Model file for the job. Use its own axes, mm. Coordinates: 2 decimals unless noted, no trailing zeros. Put each result on its own line as item: value. Start each with the question number.
Q1. Drop flat-ended pins along their axis: pin 1 (5.5 mm diameter, centred on x = 184.76, z = -85.27, fed in from +Y); pin 2 (7 mm diameter, centred on x = 306.5, z = -40, fed in from -Y); pin 3 (5.5 mm diameter, centred on x = 182.5, z = -84.5, fed in from -Y). Give the stop position or say it passes through.
Q2. Cut at A-A (y = -11). Give the number of separate pieces and of enclosed holes in the cut face, then the cut area to 3 significant figures.
Q3. Drill centre lines: line 1 along Z through (x, y) = (-194, -12.5); line 2 along X through (y, z) = (-16.75, 65.5); line 3 along X through (y, z) = (-15, 72). Where is each one in solid material? Low to high.
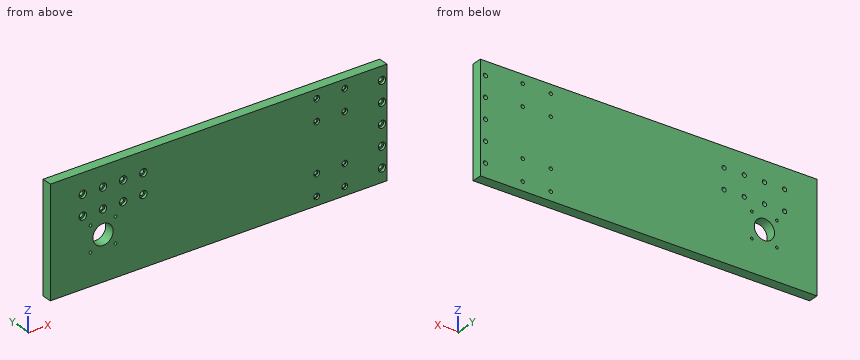
```python
from build123d import *

# Parameters (mm, degrees)
F0_W      = 635
F0_H      = 203.2
F1_DEPTH  = 19.05
F2_R      = 3.99923
F3_DEPTH  = 19.051
F4_R      = 19.05
F4_R_2    = 2.54
F5_DEPTH  = 19.051
F6_R      = 3.175
F7_DEPTH  = 19.051
F8_R      = 3.8735
F9_DEPTH  = 19.051
F10_R     = 6.985
F11_DEPTH = 4.826
F12_R     = 5.461
F13_DEPTH = 3.81


with BuildPart() as f1:
    # F0 (on Front) → F1 (new body)
    with BuildSketch(Plane.XZ):
        Rectangle(F0_W, F0_H)
    extrude(amount=F1_DEPTH)

    # F2 (on face) → F3 (cut, through all)
    with BuildSketch(Plane.XZ.offset(19.05)):
        with Locations((-256.3622, 63.8302)):
            Circle(F2_R)
        with Locations((-218.2622, 63.8302)):
            Circle(F2_R)
        with Locations((-180.1622, 63.8302)):
            Circle(F2_R)
        with Locations((-142.0622, 63.8302)):
            Circle(F2_R)
        with Locations((-142.0622, 25.7302)):
            Circle(F2_R)
        with Locations((-180.1622, 25.7302)):
            Circle(F2_R)
        with Locations((-218.2622, 25.7302)):
            Circle(F2_R)
        with Locations((-256.3622, 25.7302)):
            Circle(F2_R)
    extrude(amount=-F3_DEPTH, mode=Mode.SUBTRACT)

    # F4 (on face) → F5 (cut, through all)
    with BuildSketch(Plane.XZ.offset(19.05)):
        with Locations((-218.2622, -18.7198)):
            Circle(F4_R)
        with Locations((-241.8334, 4.8514)):
            Circle(F4_R_2)
        with Locations((-194.691, 4.8514)):
            Circle(F4_R_2)
        with Locations((-194.691, -42.291)):
            Circle(F4_R_2)
        with Locations((-241.8334, -42.291)):
            Circle(F4_R_2)
    extrude(amount=-F5_DEPTH, mode=Mode.SUBTRACT)

    # F6 (on face) → F7 (cut, through all)
    with BuildSketch(Plane.XZ.offset(19.05)):
        with Locations((184.7596, 85.2678)):
            Circle(F6_R)
        with Locations((237.7694, 85.2678)):
            Circle(F6_R)
        with Locations((184.7596, 45.2628)):
            Circle(F6_R)
        with Locations((237.7694, 45.2628)):
            Circle(F6_R)
        with Locations((184.7596, -45.2628)):
            Circle(F6_R)
        with Locations((237.7694, -45.2628)):
            Circle(F6_R)
        with Locations((184.7596, -85.2678)):
            Circle(F6_R)
        with Locations((237.7694, -85.2678)):
            Circle(F6_R)
    extrude(amount=-F7_DEPTH, mode=Mode.SUBTRACT)

    # F8 (on face) → F9 (cut, through all)
    with BuildSketch(Plane.XZ.offset(19.05)):
        with Locations((307.975, 76.2)):
            Circle(F8_R)
        with Locations((307.975, 38.1)):
            Circle(F8_R)
        with Locations((307.975, 0)):
            Circle(F8_R)
        with Locations((307.975, -38.1)):
            Circle(F8_R)
        with Locations((307.975, -76.2)):
            Circle(F8_R)
    extrude(amount=-F9_DEPTH, mode=Mode.SUBTRACT)

    # F10 (on face) → F11 (cut)
    with BuildSketch(Plane.XZ.offset(19.05)):
        with Locations((-256.3622, 63.8302)):
            Circle(F10_R)
        with Locations((-256.3622, 25.7302)):
            Circle(F10_R)
        with Locations((-218.2622, 25.7302)):
            Circle(F10_R)
        with Locations((-218.2622, 63.8302)):
            Circle(F10_R)
        with Locations((-180.1622, 63.8302)):
            Circle(F10_R)
        with Locations((-142.0622, 63.8302)):
            Circle(F10_R)
        with Locations((-180.1622, 25.7302)):
            Circle(F10_R)
        with Locations((-142.0622, 25.7302)):
            Circle(F10_R)
        with Locations((307.975, -76.2)):
            Circle(F10_R)
        with Locations((307.975, -38.1)):
            Circle(F10_R)
        with Locations((307.975, 0)):
            Circle(F10_R)
        with Locations((307.975, 38.1)):
            Circle(F10_R)
        with Locations((307.975, 76.2)):
            Circle(F10_R)
    extrude(amount=-F11_DEPTH, mode=Mode.SUBTRACT)

    # F12 (on face) → F13 (cut)
    with BuildSketch(Plane.XZ.offset(19.05)):
        with Locations((184.7596, 85.2678)):
            Circle(F12_R)
        with Locations((184.7596, 45.2628)):
            Circle(F12_R)
        with Locations((184.7596, -45.2628)):
            Circle(F12_R)
        with Locations((184.7596, -85.2678)):
            Circle(F12_R)
        with Locations((237.7694, -85.2678)):
            Circle(F12_R)
        with Locations((237.7694, -45.2628)):
            Circle(F12_R)
        with Locations((237.7694, 45.2628)):
            Circle(F12_R)
        with Locations((237.7694, 85.2678)):
            Circle(F12_R)
    extrude(amount=-F13_DEPTH, mode=Mode.SUBTRACT)


solid = f1.part
```
Computed values:
1. pin 1: through
1. pin 2: y = -14.22
1. pin 3: y = -15.24
2. separate pieces: 1
2. enclosed holes: 26
2. area: 127,000 mm2
3. line 1: -101.6 to -44.74, -39.85 to 2.41, 7.3 to 101.6
3. line 2: -317.5 to -263.14, -249.58 to -225.04, -211.48 to -186.94, -173.38 to -148.84, -135.28 to 317.5
3. line 3: -317.5 to 302.39, 313.56 to 317.5
